from build123d import *

# Parameters (mm, degrees)
CROQUIS1_W              = 70
CROQUIS1_H              = 121
SALIENTE_EXTRUIR1_DEPTH = 2
CROQUIS2_W              = 70
CROQUIS2_H              = 121
CROQUIS2_W_2            = 66
CROQUIS2_H_2            = 117
SALIENTE_EXTRUIR2_DEPTH = 22
CROQUIS3_R              = 2
CORTAR_EXTRUIR1_DEPTH   = 10


with BuildPart() as part:
    # Croquis1 → Saliente-Extruir1 (new body)
    with BuildSketch(Plane.XY):
        Rectangle(CROQUIS1_W, CROQUIS1_H)
    extrude(amount=SALIENTE_EXTRUIR1_DEPTH)

    # Croquis2 → Saliente-Extruir2 (add)
    with BuildSketch(Plane.XY.offset(2)):
        Rectangle(CROQUIS2_W, CROQUIS2_H)
        Rectangle(CROQUIS2_W_2, CROQUIS2_H_2, mode=Mode.SUBTRACT)
    extrude(amount=SALIENTE_EXTRUIR2_DEPTH)

    # Croquis3 → Cortar-Extruir1 (cut)
    with BuildSketch(Plane(origin=(0, 0, 0), x_dir=(-1, 0, 0), z_dir=(0, 0, -1))):
        with Locations((-27, 52.5)):
            Circle(CROQUIS3_R)
        with Locations((-27, -52.5)):
            Circle(CROQUIS3_R)
        with Locations((27, -52.5)):
            Circle(CROQUIS3_R)
        with Locations((27, 52.5)):
            Circle(CROQUIS3_R)
    extrude(amount=-CORTAR_EXTRUIR1_DEPTH, mode=Mode.SUBTRACT)


solid = part.part
Design review of the part built by this model. Coordinates are the model's own, in mm. A direction names the side the tool comes from. Round coordinates to 2 decimals unless told otherwise and drop trailing zeros. Loops run counter-clockwise (first coordinate to the right, second up) from the corner with the lowest first, then second, coordinate; pieces in that order, holes last. Notation, with made-up numbers: (89.5, 74.25) - (106.5, 74.25) arc R10 ccw to (106.5, 88.25) - close; hole circle Ø10 at (8, 80). An arc over 180 degrees is marked (long way). One line per question, with ' | ' between items.
1. We need section B-B, the plane z = 12.75. State the section outline as (x, y) points.
Results are:
outline: (-35, -60.5) - (35, -60.5) - (35, 60.5) - (-35, 60.5) - close; hole (-33, -58.5) - (33, -58.5) - (33, 58.5) - (-33, 58.5) - close
2. We need section A-A, the plane y = 52.5. State the section outline as (x, z) points, and give its area (3 significant figures).
Results are:
outline: (-35, 0) - (-29, 0) - (-29, 2) - (-33, 2) - (-33, 24) - (-35, 24) - close; (-25, 0) - (25, 0) - (25, 2) - (-25, 2) - close; (29, 0) - (35, 0) - (35, 24) - (33, 24) - (33, 2) - (29, 2) - close | area: 212 mm²
3. We need section D-D, the plane x = 5.5. State the section outline as (y, z) points.
Results are:
outline: (-60.5, 0) - (60.5, 0) - (60.5, 24) - (58.5, 24) - (58.5, 2) - (-58.5, 2) - (-58.5, 24) - (-60.5, 24) - close
4. For L1, parallel to Y at x = -27, z = 0.7; L2, parallel to X at y = 52, z = 18.25; L3, parallel to Y at x = 16.5, z = 2.5, list the stretches that pass through material, from the lowest coordinate up. Write a range as [from, to].
Results are:
L1: y = [-60.5, -54.5], [-50.5, 50.5], [54.5, 60.5] | L2: x = [-35, -33], [33, 35] | L3: y = [-60.5, -58.5], [58.5, 60.5]
5. We need section C-C, the plane x = -27. State the section outline as (y, z) points.
Results are:
outline: (-60.5, 0) - (-54.5, 0) - (-54.5, 2) - (-58.5, 2) - (-58.5, 24) - (-60.5, 24) - close; (-50.5, 0) - (50.5, 0) - (50.5, 2) - (-50.5, 2) - close; (54.5, 0) - (60.5, 0) - (60.5, 24) - (58.5, 24) - (58.5, 2) - (54.5, 2) - close
6. Draft analysis for pull direction Y (two halves, no side actions). For faces 1 (the face through (-27.923, -54.274, 0.986)), 2 (the face through (-35, -1, 12)), 3 (the face through (0, 1, 2)), 4 (the face through (0, 60.5, 12)), state which applies: released by +Y, released by -Y, zero draft, split by the parting line, or undercut.
Results are:
face 1: undercut | face 2: zero draft | face 3: undercut | face 4: released by +Y
7. Clearance check with flat-ended pins moving along their axes: P1, Ø5, axis at x = -27, y = 52.5, coming from the -Z side; P2, Ø3, axis at x = -18, y = 19.5, coming from the +Z side. State where each tip first meets the part, or that it passes through.
Results are:
P1: stops at z = 0 | P2: stops at z = 2
8. For faces 5 (the face through (-27.923, 50.726, 0.986)), 6 (the face through (0, 58.5, 13)), list the 3-axis set-ups (+Z, -Z, +X, -X, +Y, -Y) from which the entire face can be reached by the end or side of a thin tool; tool diameter is ignored.
Results are:
face 5: +Z, -Z | face 6: +Z
